Input: dimensioned drawing with shaded views. Units: mm. Origin: part minimum x, y, z. A direction names the side the tool comes from. Round coordinates to 2 decimals unless told otherwise and drop trailing zeros. Loops run counter-clockwise (first coordinate to the right, second up) from the corner with the lowest first, then second, coordinate; pieces in that order, holes last. Notation, with made-up numbers: M 83,20.25 L 91,20.25 A17 ccw 91,36.25 Z; hole C 75.5,46.5 d6. An arc over 180 degrees is marked long. Use one line per item in the form item = value. Start each with the question number.
Q1. Section query B-B, the plane y = 1.45. Output: boundary loops of the cut face in (x, z) (1 decimal).
Q2. Ray query, line 1 along X through (y, z) = (1.15, 2.5); line 2 along X through (y, z) = (0.85, 2); line 3 along X through (y, z) = (1.25, 8). Return the intervals inside material, ascending.
Q3. Section query D-D, the plane z = 1. Output: boundary loops of the cut face in (x, y).
Q4. Access query for the marked faces 1, 2 and 3. Directions: +Z, -Z, +X, -X, +Y, -Y. A direction counts if a zero-diameter tool reaches every point of the face in a straight line with its end or side. Return the directions, or none.
Q5. Section query C-C, the plane x = 5. Output: boundary loops of the cut face in (y, z) (1 decimal).
Q6. Mould query, pull axis X, two halves, no side actions, for the marked faces 4 and 5. Classes: pulls with the +X half, pulls with the -X half, needs draft (parallel to the pull), parting line crosses it, or undercut.
Q7. Section query A-A, the plane z = 2.5. Output: boundary loops of the cut face in (x, y).
Q8. First-contact query: P1, Ø0.5, axis at x = 11, y = 1.5, coming from the -Z side; P2, Ø0.5, axis at x = 10, y = 1, coming from the +Z side; P3, Ø3, axis at x = 11.5, z = 7.5, coming from the -Y side; P4, Ø1, axis at x = 10.5, z = 6.5, coming from the +Y side. Flat tips, straight axial feed; report the tip coordinate or a pass-through.
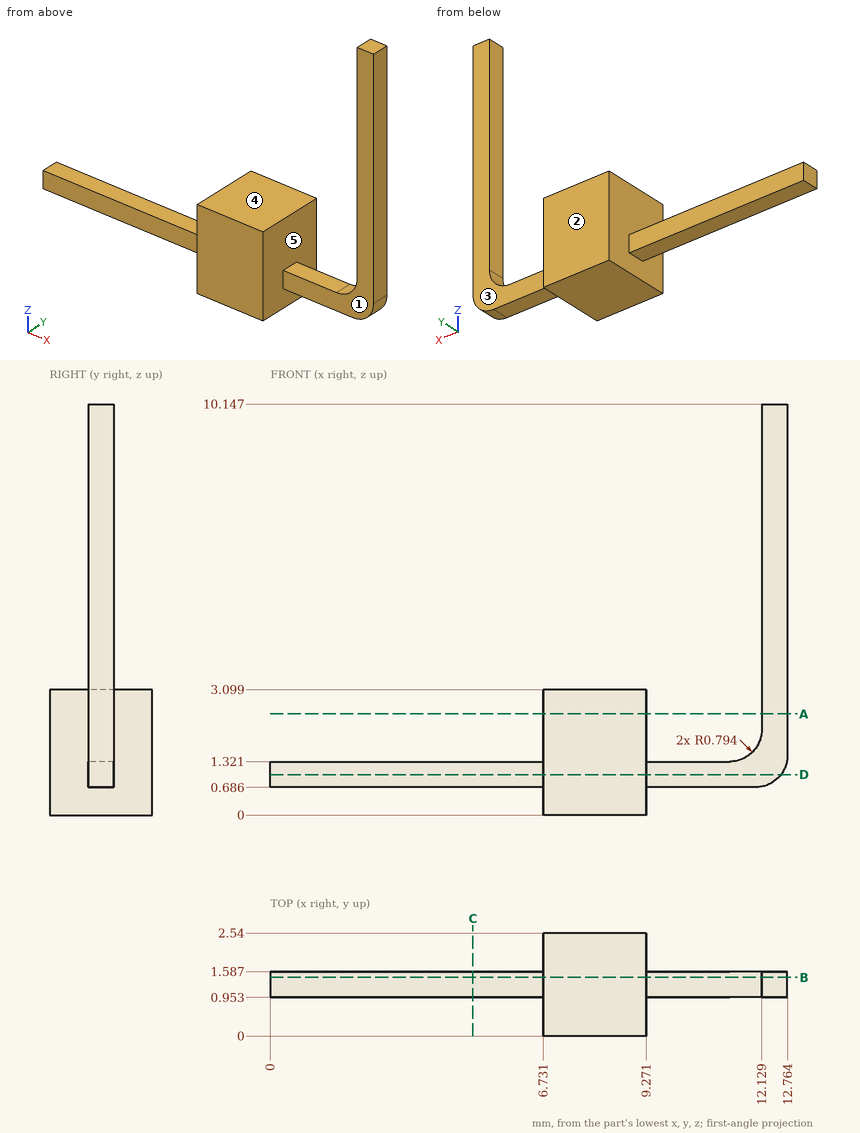
Results found:
q1.outline = M 0,0.7 L 6.7,0.7 L 6.7,0 L 9.3,0 L 9.3,0.7 L 12,0.7 A0.8 ccw 12.8,1.5 L 12.8,10.1 L 12.1,10.1 L 12.1,2.1 A0.8 cw 11.3,1.3 L 9.3,1.3 L 9.3,3.1 L 6.7,3.1 L 6.7,1.3 L 0,1.3 Z
q2.line_1 = 6.73 to 9.27, 12.13 to 12.76
q2.line_2 = 6.73 to 9.27
q2.line_3 = 12.13 to 12.76
q3.outline = M 0,0.95 L 6.73,0.95 L 6.73,0 L 9.27,0 L 9.27,0.95 L 12.6,0.95 L 12.6,1.59 L 9.27,1.59 L 9.27,2.54 L 6.73,2.54 L 6.73,1.59 L 0,1.59 Z
q4.face_1 = +Z, -Z, +X, -Y
q4.face_2 = +Z, -Z, +X, -X, +Y
q4.face_3 = +Z, -Z, +X, +Y
q5.outline = M 1,0.7 L 1.6,0.7 L 1.6,1.3 L 1,1.3 Z
q6.face_4 = needs draft
q6.face_5 = undercut
q7.outline = M 6.73,0 L 9.27,0 L 9.27,2.54 L 6.73,2.54 Z; M 12.13,0.95 L 12.76,0.95 L 12.76,1.59 L 12.13,1.59 Z
q8.P1 = 0.69
q8.P2 = 1.32
q8.P3 = 0.95
q8.P4 = through
